```python
from build123d import *

# Parameters (mm, degrees)
SKETCH1_R           = 2.38125
BOSS_EXTRUDE1_DEPTH = 12.7


with BuildPart() as part:
    # Sketch1 → Boss-Extrude1 (new body)
    with BuildSketch(Plane(origin=(0, 0, 0), x_dir=(1, 0, 0), z_dir=(0, 1, 0))):
        with BuildLine():
            Line((-17.323415526, -102.086195126), (-9.525, -94.2877796))
            ThreePointArc((-9.525, -94.2877796), (31.929749665, -82.960983237), (47.386276692, -42.8625))
            ThreePointArc((47.386276692, -42.8625), (32.081828327, -16.002591621), (1.895451068, -9.3345))
            ThreePointArc((1.895451068, -9.3345), (-9.477255338, -0.9525), (0, 9.525))
            ThreePointArc((0, 9.525), (56.473798356, -56.390420656), (-17.323415526, -102.086195126))
        make_face()
        with Locations(Location((0, 0, 0), (0, 0, 270))):
            Circle(SKETCH1_R, mode=Mode.SUBTRACT)
    extrude(amount=BOSS_EXTRUDE1_DEPTH)


solid = part.part
```
For this review, take the finished solid that the model builds, in its own axes (mm). A direction names the side the tool comes from. Round coordinates to 2 decimals unless told otherwise and drop trailing zeros. Write each loop counter-clockwise with the first axis right and the second up, starting at its lowest first coordinate (ties: lowest second). Pieces come first, ordered by that corner, then holes. Notation, with made-up numbers: M -22.5,88.25 L -14.5,88.25 A14 ccw -14.5,109.25 Z; hole C -6,84.5 d2. An arc over 180 degrees is marked long. One line per item, written item: value. Start each with the question number.
(1) Machinability: for faces 1 (the cylindrical face through (31.46, 6.26, 83.38)), 2 (the flat face through (48, 0, 43)), which of the approach directions +Z, -Z, +X, -X, +Y, -Y give a long, thin tool a straight path to every point of the face, cutting with its end or side? Answer none if there is none.
(2) We need section C-C (z = 0). Give the boundary of the cut face in (x, y) (3 decimals).
(3) Wall thickness on line 1 (Z direction, x = 2, y = 4.25); line 2 (X direction, y = 8.5, z = 0) (3 decimals); line 3 (Z direction, x = 13, y = 10.75): over which ranges is each line inside the solid? List them lowest first.
(4) We need section A-A (x = 0). Give the boundary of the cut face in (y, z) (3 decimals).
(5) Insertion check: pin 1 (7.5 mm diameter, centred on x = 0, z = 0, fed in from -Y); pin 2 (3 mm diameter, centred on x = 22, y = 8, fed in from +Z); pin 3 (1.5 mm diameter, centred on x = 45, y = 7.5, fed in from -Z); pin 4 (1.5 mm diameter, centred on x = 33.5, y = 4.5, fed in from +Z). Each pin has a flat end and moves straight along its axis. Give the tip position at first contact, or say it passes through.
(6) We need section B-B (x = 8). Give the boundary of the cut face in (y, z), and give its area (3 significant figures).
(7) The part is to be moulded in two halves that separate along Z. For faces 3 (the flat face through (-13.48, 6.26, 98.24)), 4 (the cylindrical face through (32.44, 6.26, 16.27)), 5 (the cylindrical face through (56.67, 6.26, 55.02)), say which applies: released by +Z, released by -Z, zero draft, split by the parting line, or undercut.
Result:
1. face 1: +Y, -Y
1. face 2: +Z, -Z, +X, -X, -Y
2. outline: M -9.525,0 L -2.381,0 L -2.381,12.7 L -9.525,12.7 Z; M 2.381,0 L 31.591,0 L 31.591,12.7 L 2.381,12.7 Z
3. line 1: -9.49 to -1.29, 1.29 to 9.31, 95.21 to 104.74
3. line 2: -9.525 to -2.381, 2.381 to 31.591
3. line 3: -8.03 to 8.74, 93.44 to 103.28
4. outline: M 0,-9.525 L 12.7,-9.525 L 12.7,-2.381 L 0,-2.381 Z; M 0,2.381 L 12.7,2.381 L 12.7,9.525 L 0,9.525 Z; M 0,95.25 L 12.7,95.25 L 12.7,104.775 L 0,104.775 Z
5. pin 1: y = 0
5. pin 2: z = 100.97
5. pin 3: z = 11.46
5. pin 4: z = 94.46
6. outline: M 0,-8.96 L 12.7,-8.96 L 12.7,8.6 L 0,8.6 Z; M 0,94.57 L 12.7,94.57 L 12.7,104.21 L 0,104.21 Z
6. area: 345 mm²
7. face 3: released by -Z
7. face 4: undercut
7. face 5: split by the parting line
